The model under review builds one solid part; all positions refer to its coordinate system, in mm. Face numbers are marked on the shaded views. A direction names the side the tool comes from. Round coordinates to 2 decimals unless told otherwise and drop trailing zeros. Order: outer loops, then holes, each group sorted by start corner. A loop starts at its lowest first (then second) coordinate and runs counter-clockwise, first axis right, second up. Notation, with made-up numbers: M -13,73 L 0,73 A30 ccw 0,102 Z; hole C 71.5,-38.75 d9. An arc over 180 degrees is marked long. Answer as CSV lines item,"result". Start each with the question number.
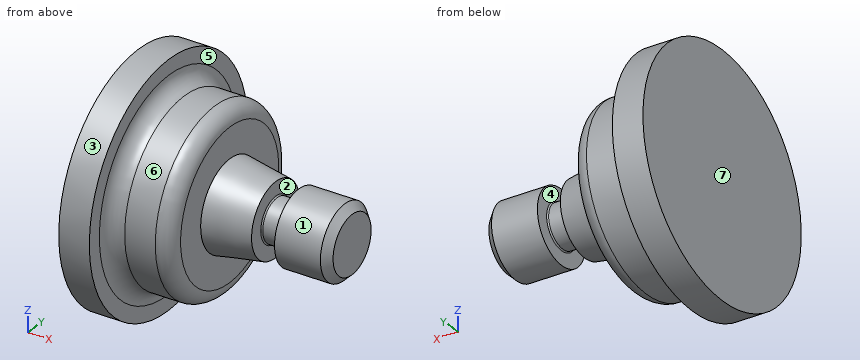
from build123d import *


with BuildPart() as part:
    # Sketch1 → Base-Revolve (revolve)
    with BuildSketch(Plane.XY, mode=Mode.PRIVATE) as base_revolve_sk:
        with BuildLine():
            Line((-88.899984186, 50.165), (-76.198738953, 50.165))
            Line((-76.198738953, 50.165), (-76.198738953, 43.815))
            ThreePointArc((-76.198738953, 43.815), (-74.339229418, 39.325746861), (-69.849976278, 37.466237326))
            Line((-69.849976278, 37.466237326), (-57.15, 37.466237326))
            ThreePointArc((-57.15, 37.466237326), (-52.658991427, 35.606000666), (-50.798754767, 31.114992093))
            Line((-50.798754767, 31.114992093), (-50.798754767, 18.414784554))
            Line((-50.798754767, 18.414784554), (-31.75, 15.239992093))
            Line((-31.75, 15.239992093), (-31.75, 9.397992093))
            ThreePointArc((-31.75, 9.397992093), (-31.601210245, 9.038781848), (-31.242, 8.889992093))
            Line((-31.242, 8.889992093), (-22.733, 8.889992093))
            ThreePointArc((-22.733, 8.889992093), (-22.373789755, 9.038781848), (-22.225, 9.397992093))
            Line((-22.225, 9.397992093), (-22.225, 15.239992093))
            Line((-22.225, 15.239992093), (-3.175, 15.239992093))
            Line((-3.175, 15.239992093), (0, 12.064992093))
            Line((0, 12.064992093), (0, 0))
            Line((0, 0), (-88.899984186, 0))
            Line((-88.899984186, 0), (-88.899984186, 50.165))
        make_face()
    revolve(base_revolve_sk.sketch.rotate(Axis((0, 0, 0), (1, 0, 0)), 90), axis=Axis((0, 0, 0), (1, 0, 0)))


solid = part.part
Item 1: For pin 1 (2 mm diameter, centred on y = -17.5, z = -32.5, fed in from +X); pin 2 (6 mm diameter, centred on x = -55, z = 24, fed in from +Y); pin 3 (5 mm diameter, centred on x = -41.5, y = -17, fed in from +Z), all flat-tipped, find the tip position at first contact; note any pin that passes through.
Item 2: Consider section C-C (x = -18). State the section outline as (y, z) points.
Item 3: Wall thickness on probe 1 along X at (y, z) = (4, 9) (3 decimals); probe 2 along X at (y, z) = (1, -27); probe 3 along Y at (x, z) = (-5, 0.5): over which ranges is each line inside the solid? List them lowest first. Write a range as [from, to].
Item 4: The part is to be moulded in two halves that separate along X. For the marked faces 4, 5, 6 and 7, say which applies: +X half, -X half, draft (parallel to the pull), parting line (faces both ways), or undercut.
Item 5: Consider section D-D (x = -64). State the section outline as (y, z) points.
Item 6: Tool access review of the marked faces 1, 2 and 3: name each direction out of +Z, -Z, +X, -X, +Y, -Y from which nothing blocks a thin tool from reaching the whole face with its end or side.
Reported:
1,pin 1,"stops at x = -52.99"
1,pin 2,"stops at y = 30.78"
1,pin 3,"stops at z = 8.69"
2,outline,"C 0,0 d30.48"
3,probe 1,"x = [-88.9, -31.75], [-22.225, 0]"
3,probe 2,"x = [-88.9, -50.8]"
3,probe 3,"y = [-15.23, 15.23]"
4,face 4,"undercut"
4,face 5,"+X half"
4,face 6,"draft"
4,face 7,"-X half"
5,outline,"C 0,0 d74.93"
6,face 1,"+X"
6,face 2,"none"
6,face 3,"+X, -X"
